The model under review builds one solid part; all positions refer to its coordinate system, in mm. A direction names the side the tool comes from. Give positions to 0.01 mm unless a question says otherwise; leave off trailing zeros. Use CSV: the item, a comma, the result in double quotes. Start each with the question number.
1. To check wall thickness, follow line 1 (Y direction, x = 3, z = 246); line 2 (X direction, y = -9.75, z = 182) (3 decimals); line 3 (Y direction, x = 10, z = 58) (3 decimals). State the ranges of each line that lie inside material, in increasing order. Write a range as [from, to].
2. For pin 1 (6 mm diameter, centred on y = -9.5, z = 173, fed in from -X); pin 2 (1.2 mm diameter, centred on y = -6, z = 98.5, fed in from +X); pin 3 (1.2 mm diameter, centred on y = -6, z = 191.5, fed in from -X), all flat-tipped, find the tip position at first contact; note any pin that passes through.
3. Draft analysis for pull direction X (two halves, no side actions). For faces 1 (the flat face through (6.175, -10, 141)), 2 (the cylindrical face through (9.72, -7.87, 140.5)), 3 (the flat face through (3, 0, 141)), state which applies: released by +X, released by -X, zero draft, split by the parting line, or undercut.
4. Machinability: for faces 4 (the flat face through (10, -13.825, 141)), 5 (the flat face through (13.825, -10, 141)), 6 (the flat face through (10, -6.175, 141)), which of the approach directions +Z, -Z, +X, -X, +Y, -Y give a long, thin tool a straight path to every point of the face, cutting with its end or side? Answer none if there is none.
```python
from build123d import *

# Parameters (mm, degrees)
CROQUIS1_R      = 2.15
BOSCHBASE_DEPTH = 285


with BuildPart() as part:
    # Croquis1 → BoschBase (new body)
    with BuildSketch(Plane.XY):
        Polygon((4.4, 0), (0, 0), (0, -0.56736664), (0, -4.4), (0, -4.95), (1.8, -6.75), (1.8, -4.4), (3.410050506, -4.4), (6.175, -7.164949494), (6.175, -12.835050506), (3.410050506, -15.6), (1.8, -15.6), (1.8, -13.25), (0, -15.05), (0, -15.6), (0, -20), (4.4, -20), (4.95, -20), (6.75, -18.2), (4.4, -18.2), (4.4, -16.589949494), (7.164949494, -13.825), (12.835050506, -13.825), (15.6, -16.589949494), (15.6, -18.2), (13.25, -18.2), (15.05, -20), (15.6, -20), (18.2, -20), (20, -20), (20, -15.6), (20, -15.05), (18.2, -13.25), (18.2, -15.6), (16.589949494, -15.6), (13.825, -12.835050506), (13.825, -7.164949494), (16.589949494, -4.4), (18.2, -4.4), (18.2, -6.75), (20, -4.95), (20, -4.4), (20, 0), (15.6, 0), (15.05, 0), (13.25, -1.8), (15.6, -1.8), (15.6, -3.410050506), (12.835050506, -6.175), (7.164949494, -6.175), (4.4, -3.410050506), (4.4, -1.8), (6.75, -1.8), (4.95, 0), align=None)
        with Locations((10, -10)):
            Circle(CROQUIS1_R, mode=Mode.SUBTRACT)
    extrude(amount=BOSCHBASE_DEPTH)


solid = part.part
```
Determined:
1,line 1,"y = [-20, -15.6], [-4.4, 0]"
1,line 2,"x = [6.175, 7.865], [12.135, 13.825]"
1,line 3,"y = [-13.825, -12.15], [-7.85, -6.175]"
2,pin 1,"stops at x = 1.55"
2,pin 2,"stops at x = 19.55"
2,pin 3,"stops at x = 0.45"
3,face 1,"released by -X"
3,face 2,"undercut"
3,face 3,"zero draft"
4,face 4,"+Z, -Z, -Y"
4,face 5,"+Z, -Z, +X"
4,face 6,"+Z, -Z, +Y"
